The model under review builds one solid part; all positions refer to its coordinate system, in mm. A direction names the side the tool comes from. Round coordinates to 2 decimals unless told otherwise and drop trailing zeros. Loops run counter-clockwise (first coordinate to the right, second up) from the corner with the lowest first, then second, coordinate; pieces in that order, holes last. Notation, with made-up numbers: (85, -25.75) -> (119, -25.75) arc R23 ccw to (119, 10.25) -> close; hole circle Ø5 at (18.25, 39). An arc over 180 degrees is marked (long way). Use CSV: the item, a comma, the result in double quotes. Start each with the question number.
```python
from build123d import *

# Parameters (mm, degrees)
SKETCH1_R               = 38.1
BOSS_EXTRUDE1_DEPTH     = 63.5
BOSS_EXTRUDE2_DEPTH     = 76.2
SKETCH3_R               = 5.08
CUT_EXTRUDE1_DEPTH      = 76.2
CUT_EXTRUDE1_DEPTH_BACK = 76.2
SKETCH4_R               = 50.8
SKETCH4_R_2             = 37.439644023
CUT_EXTRUDE4_DEPTH      = 76.2
CUT_EXTRUDE4_DEPTH_BACK = 76.2
SKETCH5_R               = 38.1
CUT_EXTRUDE8_DEPTH      = 25.4
SKETCH6_R               = 37.465
BOSS_EXTRUDE4_DEPTH     = 25.4


with BuildPart() as part:
    # Sketch1 → Boss-Extrude1 (new body)
    with BuildSketch(Plane(origin=(0, 0, 0), x_dir=(1, 0, 0), z_dir=(0, 1, 0))):
        Circle(SKETCH1_R)
    extrude(amount=BOSS_EXTRUDE1_DEPTH)

    # Sketch2 → Boss-Extrude2 (add)
    with BuildSketch(Plane(origin=(0, 0, 0), x_dir=(1, 0, 0), z_dir=(0, 1, 0))):
        with BuildLine():
            Line((-6.35, -12.7), (-6.35, 12.7))
            ThreePointArc((-6.35, 12.7), (0, 19.05), (6.35, 12.7))
            Line((6.35, 12.7), (6.35, -12.7))
            ThreePointArc((6.35, -12.7), (0, -19.05), (-6.35, -12.7))
        make_face()
    extrude(amount=BOSS_EXTRUDE2_DEPTH)

    # Sketch3 → Cut-Extrude1 (cut, two sides)
    with BuildSketch(Plane(origin=(0, 0, 0), x_dir=(0, 0, -1), z_dir=(1, 0, 0))) as cut_extrude1_sk:
        with Locations((0, 69.85)):
            Circle(SKETCH3_R)
    extrude(amount=CUT_EXTRUDE1_DEPTH, mode=Mode.SUBTRACT)
    extrude(cut_extrude1_sk.sketch, amount=-CUT_EXTRUDE1_DEPTH_BACK, mode=Mode.SUBTRACT)

    # Sketch4 → Cut-Extrude4 (cut, two sides)
    with BuildSketch(Plane(origin=(0, 0, 0), x_dir=(1, 0, 0), z_dir=(0, 1, 0))) as cut_extrude4_sk:
        Circle(SKETCH4_R)
        Circle(SKETCH4_R_2, mode=Mode.SUBTRACT)
    extrude(amount=CUT_EXTRUDE4_DEPTH, mode=Mode.SUBTRACT)
    extrude(cut_extrude4_sk.sketch, amount=-CUT_EXTRUDE4_DEPTH_BACK, mode=Mode.SUBTRACT)

    # Sketch5 → Cut-Extrude8 (cut)
    with BuildSketch(Plane(origin=(0, 76.2, 0), x_dir=(1, 0, 0), z_dir=(0, 1, 0))):
        Circle(SKETCH5_R)
        with BuildLine():
            Line((-6.341677417, -12.718199215), (-6.341677417, 12.718199215))
            ThreePointArc((-6.341677417, 12.718199215), (0, 19.059876632), (6.341677417, 12.718199215))
            Line((6.341677417, 12.718199215), (6.341677417, -12.718199215))
            ThreePointArc((6.341677417, -12.718199215), (0, -19.059876632), (-6.341677417, -12.718199215))
        make_face(mode=Mode.SUBTRACT)
    extrude(amount=-CUT_EXTRUDE8_DEPTH, mode=Mode.SUBTRACT)

    # Sketch6 → Boss-Extrude4 (add)
    with BuildSketch(Plane(origin=(0, 0, 0), x_dir=(-1, 0, 0), z_dir=(0, -1, 0))):
        Circle(SKETCH6_R)
    extrude(amount=BOSS_EXTRUDE4_DEPTH)


solid = part.part
```
1. For faces 1 (the face through (-0.1, 69.76, -19.05)), 2 (the face through (0.1, 69.76, 19.05)), 3 (the face through (-6.342, 64, 0)), 4 (the face through (6.342, 64, 0)), list the 3-axis set-ups (+Z, -Z, +X, -X, +Y, -Y) from which the entire face can be reached by the end or side of a thin tool; tool diameter is ignored.
2. Take a section at B-B, the plane y = 69.85. Give the boundary of the cut face in (x, z), then the cut area to 3 significant figures.
3. Take a section at C-C, the plane z = 0. Give the boundary of the cut face in (x, y) (3 decimals), then the cut area to 3 significant figures.
4. For line 1 along Y through (x, z) = (-0.75, 0); line 2 along X through (y, z) = (58, 0.5); line 3 along Y through (x, z) = (-3, 1), list the stretches that pass through material, from the lowest coordinate up. Write a range as from..to.
5. Clearance check with flat-ended pins moving along their axes: P1, Ø2, axis at x = 30, y = 46.5, coming from the +Z side; P2, Ø3, axis at y = 37.5, z = 11, coming from the +X side; P3, Ø1.5, axis at x = 7, y = 25, coming from the +Z side; P4, Ø6, axis at y = 69.85, z = 0, coming from the -X side. State where each tip first meets the part, or that it passes through.
6. Take a section at A-A, the plane x = 0. Give the boundary of the cut face in (y, z) (3 decimals).
7. The part is to be moulded in two halves that separate along Z. For faces 5 (the face through (1, -25.4, -1)), 6 (the face through (29.73, -12.52, 22.8)), 7 (the face through (-0.14, 58.03, -19.06)), 8 (the face through (0.09, 64.89, 1.1)), say which applies: pulls with the +Z half, pulls with the -Z half, needs draft (parallel to the pull), parting line crosses it, or undercut.
Results:
1,face 1,"-Z, +Y"
1,face 2,"+Z, +Y"
1,face 3,"+Z, -Z, -X, +Y"
1,face 4,"+Z, -Z, +X, +Y"
2,outline,"(-6.34, -12.72) arc R6.34 ccw to (-5.64, -15.61) arc R6.35 ccw to (5.64, -15.61) arc R6.34 ccw to (6.34, -12.72) -> (6.34, -5.08) -> (-6.34, -5.08) -> close; (-6.34, 5.08) -> (6.34, 5.08) -> (6.34, 12.72) arc R6.34 ccw to (5.64, 15.61) arc R6.35 ccw to (-5.64, 15.61) arc R6.34 ccw to (-6.34, 12.72) -> close"
2,area,"320 mm²"
3,outline,"(-37.465, -25.4) -> (37.465, -25.4) -> (37.465, 0) -> (37.44, 0) -> (37.44, 50.8) -> (6.342, 50.8) -> (6.342, 64.77) -> (-6.342, 64.77) -> (-6.342, 50.8) -> (-37.44, 50.8) -> (-37.44, 0) -> (-37.465, 0) -> close; (-6.342, 74.93) -> (6.342, 74.93) -> (6.342, 76.2) -> (-6.342, 76.2) -> close"
3,area,"5,900 mm²"
4,line 1,"-25.4..64.77, 74.93..76.2"
4,line 2,"-6.34..6.34"
4,line 3,"-25.4..64.87, 74.83..76.2"
5,P1,"z = 23.68"
5,P2,"x = 36.21"
5,P3,"z = 36.91"
5,P4,"through"
6,outline,"(-25.4, -37.465) -> (0, -37.465) -> (0, -37.44) -> (50.8, -37.44) -> (50.8, -19.06) -> (63.5, -19.06) -> (63.5, -19.05) -> (76.2, -19.05) -> (76.2, 19.05) -> (63.5, 19.05) -> (63.5, 19.06) -> (50.8, 19.06) -> (50.8, 37.44) -> (0, 37.44) -> (0, 37.465) -> (-25.4, 37.465) -> close; hole circle Ø10.16 at (69.85, 0)"
7,face 5,"needs draft"
7,face 6,"parting line crosses it"
7,face 7,"pulls with the -Z half"
7,face 8,"undercut"
